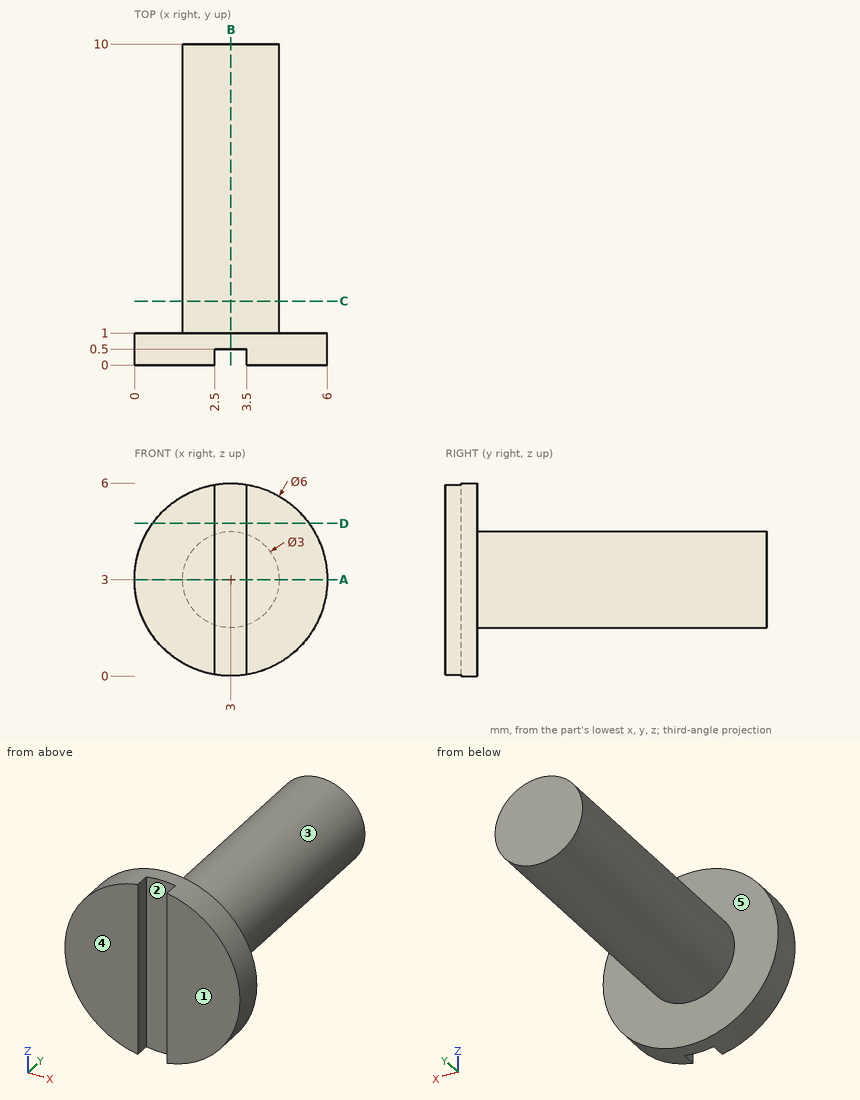
Verification items for this drawing (mm, ordinates from the low corner). A direction names the side the tool comes from. Coordinates: 2 decimals unless noted, no trailing zeros. Order: outer loops, then holes, each group sorted by start corner. A loop starts at its lowest first (then second) coordinate and runs counter-clockwise, first axis right, second up. Notation, with made-up numbers: (-1.75, -12.75) - (53.25, -12.75) arc R22 cw to (53.25, 1.25) - close; hole circle Ø6 at (72.5, 43.25). An arc over 180 degrees is marked (long way). Answer in a Markdown table with one row per item. Add a question column.
1. Section check D-D (z = 4.75). Enter the section's corners in (x, y).
2. Draft check along X on the marked faces 1, 2 and 3. Enter one of: +X half, -X half, draft (parallel to the pull), parting line (faces both ways), or undercut.
3. Section check A-A (z = 3). Enter the section's corners in (x, y), plus the area to 3 significant figures.
4. Section check B-B (x = 3). Enter the section's corners in (y, z).
5. Gauge pin test, flat ends, axial feed: pin 1 Ø1 at (x, y) = (3.5, 5) entering from -Z; pin 2 Ø3 at (y, z) = (9, 3.5) entering from -X; pin 3 Ø0.5 at (x, z) = (3, 3.5) entering from -Y. Record the tip position at first contact, or that the pin passes through.
6. Access from +Z, -Z, +X, -X, +Y, -Y to the whole of each face (thin tool, end or side, straight path). Record for the marked faces 4 and 5.
7. Material ranges on L1, parallel to Y at x = 3.2, z = 5.5; L2, parallel to Y at x = 5.35, z = 3.75; L3, parallel to Z at x = 4.3, y = 3, recorded low to high. Write a range as [from, to].
8. Section check C-C (y = 2). Enter the section's corners in (x, z).
Data:
| question | item | result |
|---|---|---|
| 1 | outline | (0.56, 0) - (2.5, 0) - (2.5, 0.5) - (3.5, 0.5) - (3.5, 0) - (5.44, 0) - (5.44, 1) - (0.56, 1) - close |
| 2 | face 1 | draft |
| 2 | face 2 | undercut |
| 2 | face 3 | parting line |
| 3 | outline | (0, 0) - (2.5, 0) - (2.5, 0.5) - (3.5, 0.5) - (3.5, 0) - (6, 0) - (6, 1) - (4.5, 1) - (4.5, 10) - (1.5, 10) - (1.5, 1) - (0, 1) - close |
| 3 | area | 32.5 mm² |
| 4 | outline | (0.5, 0) - (1, 0) - (1, 1.5) - (10, 1.5) - (10, 4.5) - (1, 4.5) - (1, 6) - (0.5, 6) - close |
| 5 | pin 1 | stops at z = 1.5 |
| 5 | pin 2 | stops at x = 1.5 |
| 5 | pin 3 | stops at y = 0.5 |
| 6 | face 4 | +Z, -Z, +X, -X, -Y |
| 6 | face 5 | +Y |
| 7 | L1 | y = [0.5, 1] |
| 7 | L2 | y = [0, 1] |
| 7 | L3 | z = [2.25, 3.75] |
| 8 | outline | circle Ø3 at (3, 3) |
